Can you work these out from the model? Positions are in its coordinate system, mm. A direction names the side the tool comes from. Coordinates: 2 decimals unless noted, no trailing zeros. Order: outer loops, then holes, each group sorted by start corner. A loop starts at its lowest first (then second) coordinate and runs counter-clockwise, first axis right, second up. Notation, with made-up numbers: (1.5, 4) -> (48.5, 4) arc R22 ccw to (48.5, 13) -> close; hole circle Ø9 at (-30.5, 67). An arc over 180 degrees is marked (long way). Answer in a Markdown table with one row per item. Add a question column.
1. Imagine slicing it at D-D on y = 16.5. Write out the boundary of the cut face in (x, z), plus the area to 3 significant figures.
2. We'd pull the mould along X, two halves only. Please class faces 1 (the face through (10, 61, 0)), 2 (the face through (20, 59, 5)), 3 (the face through (12.74, 114.3, 10.49)): pulls with the +X half, pulls with the -X half, needs draft (parallel to the pull), parting line crosses it, or undercut.
3. Imagine slicing it at A-A on y = 110. Write out the boundary of the cut face in (x, z), plus the area to 3 significant figures.
4. Imagine slicing it at B-B on x = 7.75. Write out the boundary of the cut face in (y, z), plus the area to 3 significant figures.
5. Will this pin go through, and if not, where does the flat tip stop? pin 1 (10 mm diameter, centred on x = 6.5, y = 68, fed in from +Z).
6. Imagine slicing it at C-C on z = 2.25. Write out the boundary of the cut face in (x, y), plus the area to 3 significant figures.
7. If I drill on line 1 along Y through (x, z) = (10, 3.25); line 2 along Y through (x, z) = (10, 10.3); line 3 along Y through (x, z) = (11.5, 2.25), over which ranges is the centre line in solid material (lowest first)? Write a range as [from, to].
8. On a 3-axis mill with a long thin cutter (end or side, diameter ignored), from which of +Z, -Z, +X, -X, +Y, -Y can I reach the whole of each face in a straight line? I mean faces 4 (the face through (8, 15, 11)), 5 (the face through (14.864, 11.532, 10.493)). Say none if no direction works.
from build123d import *

# Parameters (mm, degrees)
SKIZZE1_W                       = 20
SKIZZE1_H                       = 120
AUFSATZ_LINEAR_AUSTRAGEN1_DEPTH = 10
SKIZZE2_R                       = 7.5
SKIZZE2_R_2                     = 5.1
AUFSATZ_LINEAR_AUSTRAGEN3_DEPTH = 1
SKIZZE5_R                       = 5
SCHNITT_LINEAR_AUSTRAGEN1_DEPTH = 10


with BuildPart() as part:
    # Skizze1 → Aufsatz-Linear austragen1 (new body)
    with BuildSketch(Plane.XY):
        with Locations((10, 60)):
            Rectangle(SKIZZE1_W, SKIZZE1_H)
    extrude(amount=AUFSATZ_LINEAR_AUSTRAGEN1_DEPTH)

    # Skizze2 → Aufsatz-Linear austragen3 (add)
    # profile 1 of 2: a face of its own
    with BuildSketch(Plane.XY.offset(10)):
        with Locations(Location((10, 110, 0), (0, 0, 180))):
            Circle(SKIZZE2_R)
        with Locations((10, 110)):
            Circle(SKIZZE2_R_2, mode=Mode.SUBTRACT)
    # profile 2 of 2: a face of its own
    with BuildSketch(Plane.XY.offset(10)):
        with Locations(Location((10, 10, 0), (0, 0, 180))):
            Circle(SKIZZE2_R)
        with Locations((10, 10)):
            Circle(SKIZZE2_R_2, mode=Mode.SUBTRACT)
    extrude(amount=AUFSATZ_LINEAR_AUSTRAGEN3_DEPTH)

    # Skizze5 → Schnitt-Linear austragen1 (cut)
    with BuildSketch(Plane.XY.offset(10)):
        with Locations((10, 110)):
            Circle(SKIZZE5_R)
        with Locations((10, 10)):
            Circle(SKIZZE5_R)
    extrude(amount=-SCHNITT_LINEAR_AUSTRAGEN1_DEPTH, mode=Mode.SUBTRACT)


solid = part.part
Answers follow:
| question | item | result |
|---|---|---|
| 1 | outline | (0, 0) -> (20, 0) -> (20, 10) -> (13.74, 10) -> (13.74, 11) -> (6.26, 11) -> (6.26, 10) -> (0, 10) -> close |
| 1 | area | 207 mm² |
| 2 | face 1 | needs draft |
| 2 | face 2 | pulls with the +X half |
| 2 | face 3 | undercut |
| 3 | outline | (0, 0) -> (5, 0) -> (5, 10) -> (4.9, 10) -> (4.9, 11) -> (2.5, 11) -> (2.5, 10) -> (0, 10) -> close; (15, 0) -> (20, 0) -> (20, 10) -> (17.5, 10) -> (17.5, 11) -> (15.1, 11) -> (15.1, 10) -> (15, 10) -> close |
| 3 | area | 105 mm² |
| 4 | outline | (0, 0) -> (5.53, 0) -> (5.53, 10) -> (5.42, 10) -> (5.42, 11) -> (2.85, 11) -> (2.85, 10) -> (0, 10) -> close; (14.47, 0) -> (105.53, 0) -> (105.53, 10) -> (105.42, 10) -> (105.42, 11) -> (102.85, 11) -> (102.85, 10) -> (17.15, 10) -> (17.15, 11) -> (14.58, 11) -> (14.58, 10) -> (14.47, 10) -> close; (114.47, 0) -> (120, 0) -> (120, 10) -> (117.15, 10) -> (117.15, 11) -> (114.58, 11) -> (114.58, 10) -> (114.47, 10) -> close |
| 4 | area | 1,030 mm² |
| 5 | pin 1 | stops at z = 10 |
| 6 | outline | (0, 0) -> (20, 0) -> (20, 120) -> (0, 120) -> close; hole circle Ø10 at (10, 10); hole circle Ø10 at (10, 110) |
| 6 | area | 2,240 mm² |
| 7 | line 1 | y = [0, 5], [15, 105], [115, 120] |
| 7 | line 2 | y = [2.5, 4.9], [15.1, 17.5], [102.5, 104.9], [115.1, 117.5] |
| 7 | line 3 | y = [0, 5.23], [14.77, 105.23], [114.77, 120] |
| 8 | face 4 | +Z, +X, -X, +Y, -Y |
| 8 | face 5 | +Z |
